Design review of the part built by this model. Coordinates are the model's own, in mm. Coordinates: 2 decimals unless noted, no trailing zeros. Loops run counter-clockwise (first coordinate to the right, second up) from the corner with the lowest first, then second, coordinate; pieces in that order, holes last. Notation, with made-up numbers: (79, 40.5) -> (137, 40.5) arc R20 ccw to (137, 64.5) -> close; hole circle Ø9 at (-36.5, 48). An arc over 180 degrees is marked (long way). Answer in a Markdown table with one row per item.
```python
from build123d import *

# Parameters (mm, degrees)
F1_DEPTH = 3
F2_R     = 0.8
F3_W     = 4.5
F3_H     = 5
F4_DEPTH = 3.001


with BuildPart() as f1:
    # F0 (on Front) → F1 (new body)
    with BuildSketch(Plane.XZ):
        Polygon((-58.9, 0), (56, 0), (56, 19.9), (58.9, 19.9), (58.9, 40.1), (56, 40.1), (56, 60), (58.9, 60), (58.9, 80.2), (56, 80.2), (56, 100.1), (58.9, 100.1), (58.9, 120.9), (44.9, 120.9), (44.9, 118), (25, 118), (25, 120.9), (-25, 120.9), (-25, 118), (-44.9, 118), (-44.9, 120.9), (-56, 120.9), (-56, 100.1), (-58.9, 100.1), (-58.9, 79.9), (-56, 79.9), (-56, 60), (-58.9, 60), (-58.9, 39.8), (-56, 39.8), (-56, 19.9), (-58.9, 19.9), align=None)
    extrude(amount=F1_DEPTH)

    # F2
    f2_edges = [f1.edges().sort_by_distance(p)[0] for p in [
        (58.9, -1.5, 100.1),
        (58.9, -1.5, 80.2),
        (58.9, -1.5, 60),
        (58.9, -1.5, 40.1),
        (58.9, -1.5, 19.9),
        (-58.9, -1.5, 19.9),
        (-58.9, -1.5, 39.8),
        (-58.9, -1.5, 60),
        (-58.9, -1.5, 79.9),
        (-58.9, -1.5, 100.1),
        (-56, -1.5, 120.9),
        (-44.9, -1.5, 120.9),
        (-25, -1.5, 120.9),
        (25, -1.5, 120.9),
        (44.9, -1.5, 120.9),
        (58.9, -1.5, 120.9),
    ]]
    fillet(f2_edges, radius=F2_R)

    # F3 (on face) → F4 (cut, through all)
    with BuildSketch(Plane.XZ.offset(3)):
        with Locations((-37.25, 2.5)):
            Rectangle(F3_W, F3_H)
        with Locations((37.25, 2.5)):
            Rectangle(F3_W, F3_H)
    extrude(amount=-F4_DEPTH, mode=Mode.SUBTRACT)


solid = f1.part
```
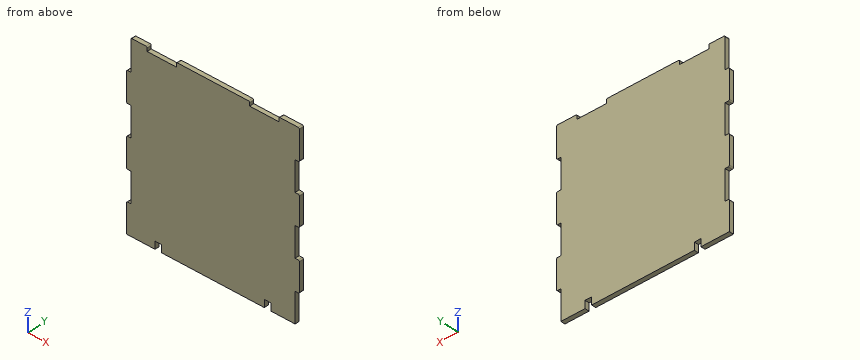
(1) Take a section at B-B on x = 37. Give the boundary of the cut face in (y, z).
Evaluation:
| item | result |
|---|---|
| outline | (-3, 5) -> (0, 5) -> (0, 118) -> (-3, 118) -> close |
(2) To check wall thickness, follow probe 1 along X at (y, z) = (-2.5, 9); probe 2 along Z at (x, y) = (-34.5, -1.7); probe 3 along X at (y, z) = (-1.85, 67). State the ranges of each line that lie inside material, in increasing order.
Evaluation:
| item | result |
|---|---|
| probe 1 | x = -58.9 to 56 |
| probe 2 | z = 0 to 118 |
| probe 3 | x = -56 to 58.9 |
(3) Take a section at A-A on z = 47. Give the boundary of the cut face in (x, y).
Evaluation:
| item | result |
|---|---|
| outline | (-58.9, -3) -> (56, -3) -> (56, 0) -> (-58.9, 0) -> close |
(4) For pin 1 (1.1 mm diameter, centred on x = 57, y = -1, fed in from -Z); pin 2 (1.5 mm diameter, centred on y = -1.5, z = 29.5, fed in from -X); pin 3 (0.6 mm diameter, centred on x = -57, y = -1.5, fed in from +Z), all flat-tipped, find the tip position at first contact; note any pin that passes through.
Evaluation:
| item | result |
|---|---|
| pin 1 | stops at z = 19.9 |
| pin 2 | stops at x = -56 |
| pin 3 | stops at z = 100.1 |
